Verification items for the finished model (mm, model axes). Give positions to 0.01 mm unless a question says otherwise; leave off trailing zeros. Order: outer loops, then holes, each group sorted by start corner. A loop starts at its lowest first (then second) coordinate and runs counter-clockwise, first axis right, second up.
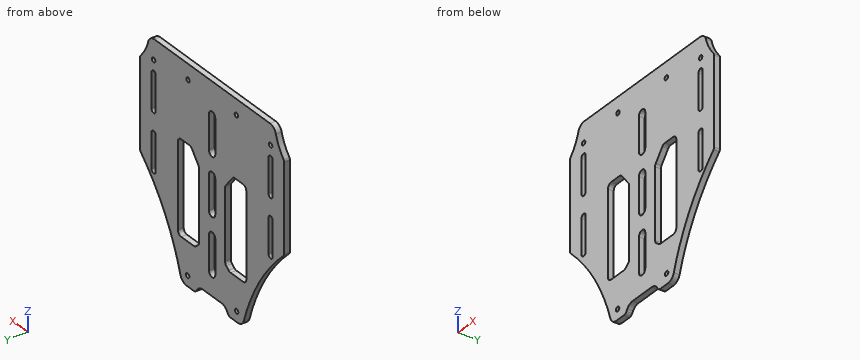
from build123d import *

# Parameters (mm, degrees)
SKETCH3_R               = 1.6
BOSS_EXTRUDE1_DEPTH     = 4
BOSS_EXTRUDE2_DEPTH     = 4
CUT_EXTRUDE1_DEPTH      = 107.208312219
CUT_EXTRUDE1_DEPTH_BACK = 107.208312219
FILLET1_R               = 2
FILLET2_R               = 2


with BuildPart() as part:
    # Sketch3 → Boss-Extrude1 (new body)
    with BuildSketch(Plane(origin=(0, 0, 0), x_dir=(1, 0, 0), z_dir=(0, 1, 0))):
        with BuildLine():
            ThreePointArc((-73.029142624, 1.757624222), (-74.485200805, -0.256695741), (-75, -2.688273856))
            Line((-75, -2.688273856), (-75, -48.998688468))
            ThreePointArc((-75, -48.998688468), (-74.409604655, -51.594103171), (-72.754607506, -53.678744287))
            add(Edge.make_bspline(
                [(-72.754607506, -53.678744287), (-69.155494376, -56.566157963), (-64.599200983, -61.832292074), (-61.843913564, -68.281231903), (-61.080449761, -70.821562762)],
                knots=[0.094602327, 0.094602327, 0.094602327, 0.094602327, 0.56783984, 0.847958174, 0.847958174, 0.847958174, 0.847958174], degree=3))
            ThreePointArc((-61.080449761, -70.821562762), (-58.914739386, -73.90928377), (-55.334342253, -75.094643974))
            Line((-55.334342253, -75.094643974), (55.334342253, -75.094643974))
            ThreePointArc((55.334342253, -75.094643974), (58.914739386, -73.90928377), (61.080449761, -70.821562762))
            add(Edge.make_bspline(
                [(72.754607506, -53.678744287), (69.155494376, -56.566157963), (64.599200983, -61.832292074), (61.843913564, -68.281231903), (61.080449761, -70.821562762)],
                knots=[0.094602327, 0.094602327, 0.094602327, 0.094602327, 0.56783984, 0.847958174, 0.847958174, 0.847958174, 0.847958174], degree=3))
            ThreePointArc((72.754607506, -53.678744287), (74.409604655, -51.594103171), (75, -48.998688468))
            Line((75, -48.998688468), (75, -2.688273856))
            ThreePointArc((75, -2.688273856), (74.485200805, -0.256695741), (73.029142624, 1.757624222))
            add(Edge.make_bspline(
                [(73.029142624, 1.757624222), (61.044308879, 12.619007824), (44.264997441, 33.305814104), (33.66455996, 57.788254978), (30.349409152, 68.542031425)],
                knots=[0.029323898, 0.029323898, 0.029323898, 0.029323898, 0.569457767, 0.950406717, 0.950406717, 0.950406717, 0.950406717], degree=3))
            ThreePointArc((30.349409152, 68.542031425), (28.179000339, 71.601741431), (24.615679564, 72.774449742))
            Line((24.615679564, 72.774449742), (17.482147291, 72.774449742))
            ThreePointArc((17.482147291, 72.774449742), (16.080583841, 72.426924039), (15.003739939, 71.464863006))
            Line((15.003739939, 71.464863006), (14.10601108, 70.148653619))
            ThreePointArc((14.10601108, 70.148653619), (11.952323278, 68.224531553), (9.149196378, 67.529480146))
            Line((9.149196378, 67.529480146), (5.71201358, 67.529480146))
            Line((5.71201358, 67.529480146), (-5.71201358, 67.529480146))
            Line((-5.71201358, 67.529480146), (-9.149196378, 67.529480146))
            ThreePointArc((-9.149196378, 67.529480146), (-11.952323278, 68.224531553), (-14.10601108, 70.148653619))
            Line((-14.10601108, 70.148653619), (-15.003739939, 71.464863006))
            ThreePointArc((-15.003739939, 71.464863006), (-16.080583841, 72.426924039), (-17.482147291, 72.774449742))
            Line((-17.482147291, 72.774449742), (-24.615679564, 72.774449742))
            ThreePointArc((-24.615679564, 72.774449742), (-28.179000339, 71.601741431), (-30.349409152, 68.542031425))
            add(Edge.make_bspline(
                [(-73.029142624, 1.757624222), (-61.044308879, 12.619007824), (-44.264997441, 33.305814104), (-33.66455996, 57.788254978), (-30.349409152, 68.542031425)],
                knots=[0.029323898, 0.029323898, 0.029323898, 0.029323898, 0.569457767, 0.950406717, 0.950406717, 0.950406717, 0.950406717], degree=3))
        make_face()
        with Locations(Location((-56, -61, 0), (0, 0, 270))):
            Circle(SKETCH3_R, mode=Mode.SUBTRACT)
        with BuildLine():
            Line((-54, -27.815735365), (-54, -52))
            ThreePointArc((-54, -52), (-56, -54), (-58, -52))
            Line((-58, -52), (-58, -27.815735365))
            ThreePointArc((-58, -27.815735365), (-56, -25.815735365), (-54, -27.815735365))
        make_face(mode=Mode.SUBTRACT)
        with Locations(Location((-23.16862443, -64.386702544, 0), (0, 0, 270))):
            Circle(SKETCH3_R, mode=Mode.SUBTRACT)
        with Locations(Location((23.16862443, -64.386702544, 0), (0, 0, 270))):
            Circle(SKETCH3_R, mode=Mode.SUBTRACT)
        with BuildLine():
            ThreePointArc((3, -52.03567912), (0, -55.03567912), (-3, -52.03567912))
            Line((-3, -52.03567912), (-3, -28.03567912))
            ThreePointArc((-3, -28.03567912), (0, -25.03567912), (3, -28.03567912))
            Line((3, -28.03567912), (3, -52.03567912))
        make_face(mode=Mode.SUBTRACT)
        with Locations(Location((56, -61, 0), (0, 0, 270))):
            Circle(SKETCH3_R, mode=Mode.SUBTRACT)
        with BuildLine():
            ThreePointArc((58, -52), (56, -54), (54, -52))
            Line((54, -52), (54, -27.815735365))
            ThreePointArc((54, -27.815735365), (56, -25.815735365), (58, -27.815735365))
            Line((58, -27.815735365), (58, -52))
        make_face(mode=Mode.SUBTRACT)
        with BuildLine():
            Line((-54, 12.184264635), (-54, -12))
            ThreePointArc((-54, -12), (-56, -14), (-58, -12))
            Line((-58, -12), (-58, 12.184264635))
            ThreePointArc((-58, 12.184264635), (-56, 14.184264635), (-54, 12.184264635))
        make_face(mode=Mode.SUBTRACT)
        with BuildLine():
            Line((-32.722260611, -18.764434552), (-32.722260611, 39.955234216))
            ThreePointArc((-32.722260611, 39.955234216), (-31.843580954, 42.07655456), (-29.722260611, 42.955234216))
            Line((-29.722260611, 42.955234216), (-17.648417807, 42.955234216))
            ThreePointArc((-17.648417807, 42.955234216), (-16.667808417, 42.790442361), (-15.794929987, 42.314171032))
            Line((-15.794929987, 42.314171032), (-13.559239731, 40.557521751))
            ThreePointArc((-13.559239731, 40.557521751), (-12.714537097, 39.509984291), (-12.412727552, 38.198584936))
            Line((-12.412727552, 38.198584936), (-12.412727552, -10.734024286))
            ThreePointArc((-12.412727552, -10.734024286), (-12.577519407, -11.714633677), (-13.053790737, -12.587512107))
            Line((-13.053790737, -12.587512107), (-19.363526346, -20.617922372))
            ThreePointArc((-19.363526346, -20.617922372), (-20.411063806, -21.462625007), (-21.722463161, -21.764434552))
            Line((-21.722463161, -21.764434552), (-29.722260611, -21.764434552))
            ThreePointArc((-29.722260611, -21.764434552), (-31.843580954, -20.885754895), (-32.722260611, -18.764434552))
        make_face(mode=Mode.SUBTRACT)
        with Locations(Location((-23.456493673, 65.613297456, 0), (0, 0, 270))):
            Circle(SKETCH3_R, mode=Mode.SUBTRACT)
        with BuildLine():
            ThreePointArc((3, -12.03567912), (0, -15.03567912), (-3, -12.03567912))
            Line((-3, -12.03567912), (-3, 11.96432088))
            ThreePointArc((-3, 11.96432088), (0, 14.96432088), (3, 11.96432088))
            Line((3, 11.96432088), (3, -12.03567912))
        make_face(mode=Mode.SUBTRACT)
        with BuildLine():
            ThreePointArc((12.412727552, 38.198584936), (12.714537097, 39.509984291), (13.559239731, 40.557521751))
            Line((13.559239731, 40.557521751), (15.794929987, 42.314171032))
            ThreePointArc((15.794929987, 42.314171032), (16.667808417, 42.790442361), (17.648417807, 42.955234216))
            Line((17.648417807, 42.955234216), (29.722260611, 42.955234216))
            ThreePointArc((29.722260611, 42.955234216), (31.843580954, 42.07655456), (32.722260611, 39.955234216))
            Line((32.722260611, 39.955234216), (32.722260611, -18.764434552))
            ThreePointArc((32.722260611, -18.764434552), (31.843580954, -20.885754895), (29.722260611, -21.764434552))
            Line((29.722260611, -21.764434552), (21.722463161, -21.764434552))
            ThreePointArc((21.722463161, -21.764434552), (20.411063806, -21.462625007), (19.363526346, -20.617922372))
            Line((19.363526346, -20.617922372), (13.053790737, -12.587512107))
            ThreePointArc((13.053790737, -12.587512107), (12.577519407, -11.714633677), (12.412727552, -10.734024286))
            Line((12.412727552, -10.734024286), (12.412727552, 38.198584936))
        make_face(mode=Mode.SUBTRACT)
        with BuildLine():
            ThreePointArc((58, -12), (56, -14), (54, -12))
            Line((54, -12), (54, 12.184264635))
            ThreePointArc((54, 12.184264635), (56, 14.184264635), (58, 12.184264635))
            Line((58, 12.184264635), (58, -12))
        make_face(mode=Mode.SUBTRACT)
        with BuildLine():
            ThreePointArc((3, 27.96432088), (0, 24.96432088), (-3, 27.96432088))
            Line((-3, 27.96432088), (-3, 51.96432088))
            ThreePointArc((-3, 51.96432088), (0, 54.96432088), (3, 51.96432088))
            Line((3, 51.96432088), (3, 27.96432088))
        make_face(mode=Mode.SUBTRACT)
        with Locations(Location((16, 54.96432088, 0), (0, 0, 270))):
            Circle(SKETCH3_R, mode=Mode.SUBTRACT)
        with Locations(Location((23.456493673, 65.613297456, 0), (0, 0, 270))):
            Circle(SKETCH3_R, mode=Mode.SUBTRACT)
    extrude(amount=BOSS_EXTRUDE1_DEPTH)

    # Sketch5 → Boss-Extrude2 (add)
    with BuildSketch(Plane(origin=(0, 4, 0), x_dir=(1, 0, 0), z_dir=(0, 1, 0))):
        Polygon((15.245312242, 58.61530822), (12.156907233, 54.222909984), (18.333717252, 47.016631629), (24.002436461, 55.07881006), align=None)
    extrude(amount=-BOSS_EXTRUDE2_DEPTH)

    # Sketch7 → Cut-Extrude1 (cut, two sides: drawn at the far end of the back side and taken through both)
    with BuildSketch(Plane(origin=(0, 4, 0), x_dir=(1, 0, 0), z_dir=(0, 1, 0)).offset(-CUT_EXTRUDE1_DEPTH_BACK)):
        with BuildLine():
            ThreePointArc((-75, -48.998688468), (-74.409604655, -51.594103171), (-72.754607506, -53.678744287))
            add(Edge.make_bspline(
                [(-72.754607506, -53.678744287), (-71.398986726, -54.766300537), (-70.147919267, -55.913530515), (-69, -57.122898046)],
                knots=[0.094602327, 0.094602327, 0.094602327, 0.094602327, 0.272849185, 0.272849185, 0.272849185, 0.272849185], degree=3))
            Line((-69, -57.122898046), (-69, 5.535291358))
            add(Edge.make_bspline(
                [(-73.029142624, 1.757624222), (-71.658027629, 3.000211832), (-70.314990302, 4.259416425), (-69, 5.535291358)],
                knots=[0.029323898, 0.029323898, 0.029323898, 0.029323898, 0.091117467, 0.091117467, 0.091117467, 0.091117467], degree=3))
            ThreePointArc((-73.029142624, 1.757624222), (-74.485200805, -0.256695741), (-75, -2.688273856))
            Line((-75, -2.688273856), (-75, -48.998688468))
        make_face()
        with BuildLine():
            Line((69, 5.535291358), (69, -57.122898046))
            add(Edge.make_bspline(
                [(69, -57.122898046), (70.147919267, -55.913530515), (71.398986726, -54.766300537), (72.754607506, -53.678744287)],
                knots=[0.669711316, 0.669711316, 0.669711316, 0.669711316, 0.847958174, 0.847958174, 0.847958174, 0.847958174], degree=3))
            ThreePointArc((72.754607506, -53.678744287), (74.409604655, -51.594103171), (75, -48.998688468))
            Line((75, -48.998688468), (75, -2.688273856))
            ThreePointArc((75, -2.688273856), (74.485200805, -0.256695741), (73.029142624, 1.757624222))
            add(Edge.make_bspline(
                [(73.029142624, 1.757624222), (71.658027629, 3.000211832), (70.314990302, 4.259416425), (69, 5.535291358)],
                knots=[0.029323898, 0.029323898, 0.029323898, 0.029323898, 0.091117467, 0.091117467, 0.091117467, 0.091117467], degree=3))
        make_face()
    extrude(amount=CUT_EXTRUDE1_DEPTH + CUT_EXTRUDE1_DEPTH_BACK, mode=Mode.SUBTRACT)

    # Fillet1
    fillet1_edges = [part.edges().sort_by_distance(p)[0] for p in [
        (-69, 2, -5.535291358),
    ]]
    fillet(fillet1_edges, radius=FILLET1_R)

    # Fillet2
    fillet2_edges = [part.edges().sort_by_distance(p)[0] for p in [
        (-69, 2, 57.122898046),
        (69, 2, 57.122898046),
        (69, 2, -5.535291358),
    ]]
    fillet(fillet2_edges, radius=FILLET2_R)


solid = part.part
(1) Go/stop test with flat-tipped pins: pin 1 (2 mm diameter, centred on y = 2.5, z = -37, fed in from -X); pin 2 (1.2 mm diameter, centred on y = 2.5, z = -25.5, fed in from +X). Record where each tip stops, or that it passes through.
Solved:
pin 1: stops at x = -44.77
pin 2: stops at x = 52.12
(2) Scan lines: line 1 (X direction, y = 2.8, z = 0); line 2 (X direction, y = 1.85, z = 38.5); line 3 (X direction, y = 2.2, z = 61). Record each from-to range of solid material in increasing order.
Solved:
line 1: x = -69 to -58, -54 to -32.72, -12.41 to -3, 3 to 12.41, 32.72 to 54, 58 to 69
line 2: x = -69 to -58, -54 to -3, 3 to 54, 58 to 69
line 3: x = -65.82 to -57.6, -54.4 to 54.4, 57.6 to 65.82
(3) Section check B-B, the plane z = -9.5. Give the number of separate pieces and of enclosed holes in the cut face, then the cut area to 3 significant figures.
Solved:
separate pieces: 6
enclosed holes: 0
area: 302 mm2
(4) Section check A-A, the plane z = 48.5. Enter the section's corners in (x, y).
Solved:
outline: (-69, 0) - (-58, 0) - (-58, 4) - (-69, 4) - close; (-54, 0) - (-3, 0) - (-3, 4) - (-54, 4) - close; (3, 0) - (54, 0) - (54, 4) - (3, 4) - close; (58, 0) - (69, 0) - (69, 4) - (58, 4) - close
